```python
from build123d import *

# Parameters (mm, degrees)
SKETCH_1_W          = 63
SKETCH_1_H          = 62
EXTRUDE_1_DEPTH     = 3
SKETCH_2_W          = 25.15
SKETCH_2_H          = 62
SKETCH_2_R          = 1.65
EXTRUDE_2_DEPTH     = 12
CUT_EXTRUDE_START   = -45
SKETCH_4_R          = 1.65
SKETCH_4_W          = 22.15
SKETCH_4_H          = 41
CUT_EXTRUDE_4_DEPTH = 45
FILLET_1_R          = 1
FILLET_2_R          = 5
SKETCH_5_W          = 20.15
SKETCH_5_H          = 9
CUT_EXTRUDE_5_DEPTH = 70
FILLET_3_R          = 3
FILLET_4_R          = 3


with BuildPart() as part:
    # 草图1 → 凸台-拉伸1 (new body)
    with BuildSketch(Plane.XY):
        with Locations((3.5, -25)):
            Rectangle(SKETCH_1_W, SKETCH_1_H)
        with BuildLine():
            Line((26.8, 0), (26.8, -50))
            ThreePointArc((26.8, -50), (29, -52.2), (31.2, -50))
            Line((31.2, -50), (31.2, 0))
            ThreePointArc((31.2, 0), (29, 2.2), (26.8, 0))
        make_face(mode=Mode.SUBTRACT)
        with BuildLine():
            Line((-23.2, 0), (-23.2, -50))
            ThreePointArc((-23.2, -50), (-21, -52.2), (-18.8, -50))
            Line((-18.8, -50), (-18.8, 0))
            ThreePointArc((-18.8, 0), (-21, 2.2), (-23.2, 0))
        make_face(mode=Mode.SUBTRACT)
    extrude(amount=EXTRUDE_1_DEPTH)

    # 草图2 → 凸台-拉伸2 (add)
    with BuildSketch(Plane.XY.offset(3)):
        with Locations((10.425, -25)):
            Rectangle(SKETCH_2_W, SKETCH_2_H)
        with Locations((5.7, -1)):
            Circle(SKETCH_2_R, mode=Mode.SUBTRACT)
        with Locations((15.7, -1)):
            Circle(SKETCH_2_R, mode=Mode.SUBTRACT)
        with Locations((15.7, -49)):
            Circle(SKETCH_2_R, mode=Mode.SUBTRACT)
        with Locations((5.7, -49)):
            Circle(SKETCH_2_R, mode=Mode.SUBTRACT)
    extrude(amount=EXTRUDE_2_DEPTH)

    # 草图4 → 切除-拉伸4 (cut)
    with BuildSketch(Plane.XY.offset(15).offset(CUT_EXTRUDE_START)):
        with Locations((5.7, -1)):
            Circle(SKETCH_4_R)
        with Locations((5.7, -49)):
            Circle(SKETCH_4_R)
        with Locations((15.7, -49)):
            Circle(SKETCH_4_R)
        with Locations((15.7, -1)):
            Circle(SKETCH_4_R)
        with Locations((10.425, -25)):
            Rectangle(SKETCH_4_W, SKETCH_4_H)
    extrude(amount=CUT_EXTRUDE_4_DEPTH, mode=Mode.SUBTRACT)

    # 圆角1
    fillet_1_edges = [part.edges().sort_by_distance(p)[0] for p in [
        (-2.15, 6, 9),
        (-2.15, -56, 9),
        (23, -56, 9),
        (23, 6, 9),
        (-28, 6, 1.5),
        (35, 6, 1.5),
        (35, -56, 1.5),
        (-28, -56, 1.5),
    ]]
    fillet(fillet_1_edges, radius=FILLET_1_R)

    # 圆角2
    # the kernel refuses this fillet: 5 mm, written as the material it adds along each edge
    with BuildSketch(Plane(origin=(-2.15, -55, 3), x_dir=(0, 0, 1), z_dir=(0, 1, 0))) as fillet_2_piece_1:
        with BuildLine():
            CenterArc((FILLET_2_R, -FILLET_2_R), FILLET_2_R, 90, 90)
            Line((0, -FILLET_2_R), (0, 0))
            Line((0, 0), (FILLET_2_R, 0))
        make_face()
    extrude(amount=60)
    with BuildSketch(Plane(origin=(-1.15, 5, 3), x_dir=(-0.9999802608561372, -0.006283143965558402, 0), z_dir=(-0.006283143965558402, 0.9999802608561372, 0))) as fillet_2_piece_2_section:
        with BuildLine():
            CenterArc((-1 - FILLET_2_R, FILLET_2_R), FILLET_2_R, 270, 90)
            Line((-1 - FILLET_2_R, 0), (-1, 0))
            Line((-1, 0), (-1, FILLET_2_R))
        make_face()
    fillet_2_piece_2 = revolve(axis=Axis((-1.15, 5, 3), (0, 0, 1)), revolution_arc=359.64, mode=Mode.PRIVATE)
    fillet_2_piece_2 = split(fillet_2_piece_2, bisect_by=Plane(origin=(-1.917475009, 6, 5.017645476), z_dir=(0, -1, 0)), keep=Keep.TOP, mode=Mode.PRIVATE)
    add(fillet_2_piece_2)
    with BuildSketch(Plane(origin=(-1.15, -55, 3), x_dir=(-0.9999802608561372, 0.006283143965561067, 0), z_dir=(-0.006283143965561067, -0.9999802608561372, 0))) as fillet_2_piece_3_section:
        with BuildLine():
            CenterArc((-1 - FILLET_2_R, -FILLET_2_R), FILLET_2_R, 0, 90)
            Line((-1 - FILLET_2_R, 0), (-1, 0))
            Line((-1, 0), (-1, -FILLET_2_R))
        make_face()
    fillet_2_piece_3 = revolve(axis=Axis((-1.15, -55, 3), (0, 0, -1)), revolution_arc=359.64, mode=Mode.PRIVATE)
    fillet_2_piece_3 = split(fillet_2_piece_3, bisect_by=Plane(origin=(-1.917475041, -56, 5.017645533), z_dir=(0, 1, 0)), keep=Keep.TOP, mode=Mode.PRIVATE)
    add(fillet_2_piece_3)

    # 草图5 → 切除-拉伸5 (cut)
    with BuildSketch(Plane(origin=(0, -56, 0), x_dir=(-1, 0, 0), z_dir=(0, -1, 0))):
        with Locations((-10.925, -7.5)):
            Rectangle(SKETCH_5_W, SKETCH_5_H)
    extrude(amount=-CUT_EXTRUDE_5_DEPTH, mode=Mode.SUBTRACT)

    # 圆角3
    fillet_3_edges = [part.edges().sort_by_distance(p)[0] for p in [
        (0.85, 0.75, 3),
        (0.85, -50.75, 3),
        (21, 0.75, 3),
        (21, -50.75, 3),
    ]]
    fillet(fillet_3_edges, radius=FILLET_3_R)

    # 圆角4
    # the kernel refuses this fillet: 3 mm, written as the material it adds along each edge
    with BuildSketch(Plane(origin=(23, 5, 3), x_dir=(1, 0, 0), z_dir=(0, -1, 0))) as fillet_4_piece_1:
        with BuildLine():
            CenterArc((FILLET_4_R, FILLET_4_R), FILLET_4_R, 180, 90)
            Line((0, FILLET_4_R), (0, 0))
            Line((0, 0), (FILLET_4_R, 0))
        make_face()
    extrude(amount=60)
    with BuildSketch(Plane(origin=(22, 5, 3), x_dir=(0.9999802608561372, -0.0062831439655584, 0), z_dir=(0.0062831439655584, 0.9999802608561372, 0))) as fillet_4_piece_2_section:
        with BuildLine():
            CenterArc((-1 - FILLET_4_R, -FILLET_4_R), FILLET_4_R, 0, 90)
            Line((-1, -FILLET_4_R), (-1, 0))
            Line((-1, 0), (-1 - FILLET_4_R, 0))
        make_face()
    fillet_4_piece_2 = revolve(axis=Axis((22, 5, 3), (0, 0, -1)), revolution_arc=359.64, mode=Mode.PRIVATE)
    fillet_4_piece_2 = split(fillet_4_piece_2, bisect_by=Plane(origin=(22.764056834, 6, 4.135633635), z_dir=(0, -1, 0)), keep=Keep.TOP, mode=Mode.PRIVATE)
    add(fillet_4_piece_2)
    with BuildSketch(Plane(origin=(22, -55, 3), x_dir=(0.9999802608561372, 0.006283143965561065, 0), z_dir=(0.006283143965561065, -0.9999802608561372, 0))) as fillet_4_piece_3_section:
        with BuildLine():
            CenterArc((-1 - FILLET_4_R, FILLET_4_R), FILLET_4_R, 270, 90)
            Line((-1 - FILLET_4_R, 0), (-1, 0))
            Line((-1, 0), (-1, FILLET_4_R))
        make_face()
    fillet_4_piece_3 = revolve(axis=Axis((22, -55, 3), (0, 0, 1)), revolution_arc=359.64, mode=Mode.PRIVATE)
    fillet_4_piece_3 = split(fillet_4_piece_3, bisect_by=Plane(origin=(22.76405677, -56, 4.135633616), z_dir=(0, 1, 0)), keep=Keep.TOP, mode=Mode.PRIVATE)
    add(fillet_4_piece_3)


solid = part.part
```
Verification items for the finished model (mm, model axes). A direction names the side the tool comes from. Coordinates: 2 decimals unless noted, no trailing zeros. Order: outer loops, then holes, each group sorted by start corner. A loop starts at its lowest first (then second) coordinate and runs counter-clockwise, first axis right, second up. Notation, with made-up numbers: (62, 61.5) - (85, 61.5) arc R17 ccw to (85, 83.5) - close; hole circle Ø1 at (-32.75, -28). An arc over 180 degrees is marked (long way). Return JSON: item names as keys, results as strings.
(1) Section check A-A, the plane z = 9. Record the cut outline in (x, y), and give its area (3 significant figures).
Filled sheet:
{"outline": "(-2.15, -55) arc R1 ccw to (-1.15, -56) - (0.85, -56) - (0.85, -45.5) - (-0.65, -45.5) - (-0.65, -4.5) - (0.85, -4.5) - (0.85, 6) - (-1.15, 6) arc R1 ccw to (-2.15, 5) - close; (21, -56) - (22, -56) arc R1 ccw to (23, -55) - (23, 5) arc R1 ccw to (22, 6) - (21, 6) - (21, -4.5) - (21.5, -4.5) - (21.5, -45.5) - (21, -45.5) - close", "area": "227 mm^2"}
(2) Access from +Z, -Z, +X, -X, +Y, -Y to the whole of each face (thin tool, end or side, straight path). Record for faces 4 (the flat face through (23, -25, 10)), 5 (the flat face through (10, -45.5, 2)), 6 (the flat face through (21, 1, 9)).
Filled sheet:
{"face 4": "+Z, +X, +Y, -Y", "face 5": "+Z, -Z", "face 6": "+Y, -Y"}
(3) Section check B-B, the plane y = -39. Record the cut outline in (x, z).
Filled sheet:
{"outline": "(-28, 0) - (-23.2, 0) - (-23.2, 3) - (-28, 3) - close; (-18.8, 0) - (-0.65, 0) - (-0.65, 15) - (-2.15, 15) - (-2.15, 8) arc R5 cw to (-7.15, 3) - (-18.8, 3) - close; (21.5, 0) - (26.8, 0) - (26.8, 3) - (26, 3) arc R3 cw to (23, 6) - (23, 15) - (21.5, 15) - close; (31.2, 0) - (35, 0) - (35, 3) - (31.2, 3) - close"}
(4) Go/stop test with flat-tipped pins: pin 1 (2.5 mm diameter, centred on x = 15.7, y = -49, fed in from +Z); pin 2 (6.5 mm diameter, centred on y = -49, z = 10.5, fed in from +X); pin 3 (2 mm diameter, centred on y = -19, z = 13.5, fed in from -X); pin 4 (6.5 mm diameter, centred on y = -52, z = 10, fed in from -X). Record where each tip stops, or that it passes through.
Filled sheet:
{"pin 1": "passes through", "pin 2": "stops at x = 23", "pin 3": "stops at x = -2.15", "pin 4": "stops at x = -2.31"}
(5) Section check C-C, the plane x = 5.7. Give the number of separate pieces and of enclosed holes in the cut face, and give its area (3 significant figures).
Filled sheet:
{"separate pieces": "8", "enclosed holes": "0", "area": "86.4 mm^2"}
(6) Mould release check, pull along Y, two halves, no side actions. Record for faces 1 (the flat face through (11, -51, 12)), 2 (the cylindrical face through (29, 2.2, 1.5)), 3 (the flat face through (6, 6, 2)): pulls with the +Y half, pulls with the -Y half, needs draft (parallel to the pull), parting line crosses it, or undercut.
Filled sheet:
{"face 1": "needs draft", "face 2": "undercut", "face 3": "pulls with the +Y half"}
(7) Section check D-D, the plane x = 29. Record the cut outline in (y, z).
Filled sheet:
{"outline": "(-56, 0) - (-52.2, 0) - (-52.2, 3) - (-56, 3) - close; (2.2, 0) - (6, 0) - (6, 3) - (2.2, 3) - close"}
(8) Thickness scan on line 1 along Y through (x, z) = (5.7, 13.8); line 2 along X through (y, z) = (-49, 2.2); line 3 along X through (y, z) = (-49, 13.15). Record the ranges inside material, lowest first.
Filled sheet:
{"line 1": "y = -56 to -50.65, -47.35 to -45.5, -4.5 to -2.65, 0.65 to 6", "line 2": "x = -28 to -23.2, -18.8 to 4.05, 7.35 to 14.05, 17.35 to 26.8, 31.2 to 35", "line 3": "x = -2.15 to 4.05, 7.35 to 14.05, 17.35 to 23"}
